Design review of the part built by this model. Coordinates are the model's own, in mm. Face numbers are marked on the shaded views. A direction names the side the tool comes from. Coordinates: 2 decimals unless noted, no trailing zeros. Loops run counter-clockwise (first coordinate to the right, second up) from the corner with the lowest first, then second, coordinate; pieces in that order, holes last.
Q1. Add section D-D on x = 1.85. Give the boundary of the cut face in (y, z).
Q2. Machinability: for the marked faces 1 and 2, which of the approach directions +Z, -Z, +X, -X, +Y, -Y give a long, thin tool a straight path to every point of the face, cutting with its end or side? Answer none if there is none.
Q3. Wall thickness on probe 1 along Y at (x, z) = (-1.2, 1); probe 2 along Z at (x, y) = (-1.4, -4.25); probe 3 along X at (y, z) = (3, 1.5): over which ranges is each line inside the solid? List them lowest first.
Q4. For P1, Ø3, axis at y = 1.5, z = -1, coming from the -X side, flat-tipped, find the tip position at first contact; note if it passes through.
Q5. Add section B-B on y = 4.5. Give the boundary of the cut face in (x, z).
Q6. Add section A-A on x = -1.2. Give the boundary of the cut face in (y, z).
Q7. Add section C-C on z = 0.25. Give the boundary of the cut face in (x, y).
Q8. Draft analysis for pull direction Z (two halves, no side actions). For the marked faces 3, 4 and 5, state which applies: released by +Z, released by -Z, zero draft, split by the parting line, or undercut.
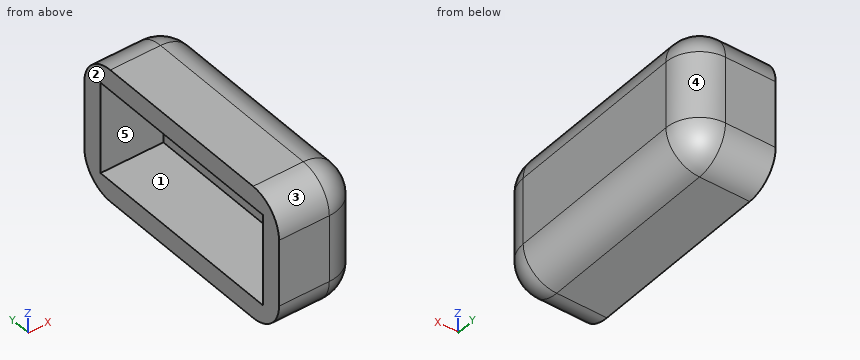
```python
from build123d import *

# Parameters (mm, degrees)
F0_W     = 15
F0_H     = 8
F1_DEPTH = 2.5
F2_T     = -1.25
F3_R     = 2


# Not quite as in the source:
# - a feature names something its author has since deleted; it is built from what else it names


with BuildPart() as f1:
    # F0 (on Right) → F1 (new body, symmetric)
    with BuildSketch(Plane.YZ):
        Rectangle(F0_W, F0_H)
    extrude(amount=F1_DEPTH, both=True)

    # F2
    f2_openings = [f1.faces().sort_by_distance(p)[0] for p in [
        (-2.5, 0, 0),
    ]]
    offset(amount=F2_T, openings=f2_openings)

    # F3
    f3_edges = [f1.edges().sort_by_distance(p)[0] for p in [
        (2.5, 0, 4),
        (2.5, -7.5, 0),
        (2.5, 0, -4),
        (2.5, 7.5, 0),
        (0, -7.5, 4),
        (0, 7.5, 4),
        (0, 7.5, -4),
        (0, -7.5, -4),
    ]]
    fillet(f3_edges, radius=F3_R)


solid = f1.part
```
Entries:
1. outline: (-6.98, -2) arc R1.48 ccw to (-5.5, -3.48) - (5.5, -3.48) arc R1.48 ccw to (6.98, -2) - (6.98, 2) arc R1.48 ccw to (5.5, 3.48) - (-5.5, 3.48) arc R1.48 ccw to (-6.98, 2) - close
2. face 1: -X
2. face 2: +Z, -Z, -X, +Y, -Y
3. probe 1: y = -7.5 to -6.25, 6.25 to 7.5
3. probe 2: z = -4 to -2.75, 2.75 to 4
3. probe 3: x = 1.25 to 2.5
4. P1: stops at x = 1.25
5. outline: (-2.5, -4) - (0.5, -4) arc R2 ccw to (2.5, -2) - (2.5, 2) arc R2 ccw to (0.5, 4) - (-2.5, 4) - (-2.5, 2.75) - (1.25, 2.75) - (1.25, -2.75) - (-2.5, -2.75) - close
6. outline: (-7.5, -2) arc R2 ccw to (-5.5, -4) - (5.5, -4) arc R2 ccw to (7.5, -2) - (7.5, 2) arc R2 ccw to (5.5, 4) - (-5.5, 4) arc R2 ccw to (-7.5, 2) - close; hole (-6.25, -2.75) - (6.25, -2.75) - (6.25, 2.75) - (-6.25, 2.75) - close
7. outline: (-2.5, -7.5) - (0.5, -7.5) arc R2 ccw to (2.5, -5.5) - (2.5, 5.5) arc R2 ccw to (0.5, 7.5) - (-2.5, 7.5) - (-2.5, 6.25) - (1.25, 6.25) - (1.25, -6.25) - (-2.5, -6.25) - close
8. face 3: released by +Z
8. face 4: zero draft
8. face 5: undercut
